Work out the finished part from the listing and answer in its coordinate system (mm). A direction names the side the tool comes from. Round coordinates to 2 decimals unless told otherwise and drop trailing zeros. Order: outer loops, then holes, each group sorted by start corner. A loop starts at its lowest first (then second) coordinate and runs counter-clockwise, first axis right, second up. Notation, with made-up numbers: (85.5, 23.5) -> (102.5, 23.5) arc R13 cw to (102.5, 43.5) -> close; hole circle Ø3 at (-38, 62.25). An arc over 180 degrees is marked (long way). Use a Markdown table: item, result. Add a question column.
Item 1: Find the intervals of material crossed by L1, parallel to Z at x = -2, y = 1.5; L2, parallel to X at y = -2.25, z = 21.5; L3, parallel to Y at x = -2, z = 27, in increasing order. Write a range as [from, to].
Item 2: A tool of negligible diameter and unlimited length cuts with its end or side. For faces 1 (the flat face through (-1.6, -1.4, 0)), 2 (the flat face through (-3.919, 0, 15)), 3 (the cylindrical face through (0.512, 0.583, 32.958)), from which of +Z, -Z, +X, -X, +Y, -Y can it reach the whole face along a straight path? Write none if from no direction.
Item 3: A cutting plane is placed at B-B, the plane y = -0.75. Determine the outline of the cut face in (x, z).
Item 4: A cutting plane is placed at C-C, the plane x = -1.5. Determine the outline of the cut face in (y, z), plus the area to 3 significant figures.
Item 5: A cutting plane is placed at D-D, the plane y = 2.25. Determine the outline of the cut face in (x, z), plus the area to 3 significant figures.
Item 6: A cutting plane is placed at A-A, the plane z = 3. Determine the outline of the cut face in (x, y).
from build123d import *

# Parameters (mm, degrees)
BOSS_EXTRUDE1_DEPTH = 30
SKETCH2_R           = 1.5
BOSS_EXTRUDE2_DEPTH = 6
SKETCH3_R           = 1.5
BOSS_EXTRUDE3_DEPTH = 6


with BuildPart() as part:
    # Sketch1 → Boss-Extrude1 (new body)
    with BuildSketch(Plane.XY):
        Polygon((-0.918598934, -3.331524887), (2.081401066, -1.599474079), (2.081401066, 1.864627536), (-0.918598934, 3.596678344), (-3.918598934, 1.864627536), (-3.918598934, -1.599474079), align=None)
    extrude(amount=BOSS_EXTRUDE1_DEPTH)

    # Sketch2 → Boss-Extrude2 (add)
    with BuildSketch(Plane.XY.offset(30)):
        with Locations((-0.918598934, 0.132576728)):
            Circle(SKETCH2_R)
    extrude(amount=BOSS_EXTRUDE2_DEPTH)

    # Sketch3 → Boss-Extrude3 (add)
    with BuildSketch(Plane(origin=(0, 0, 0), x_dir=(-1, 0, 0), z_dir=(0, 0, -1))):
        with Locations((0.918598934, 0.132576728)):
            Circle(SKETCH3_R)
    extrude(amount=BOSS_EXTRUDE3_DEPTH)


solid = part.part
Reported:
| question | item | result |
|---|---|---|
| 1 | L1 | [0, 30] |
| 1 | L2 | [-2.79, 0.95] |
| 1 | L3 | [-2.71, 2.97] |
| 2 | face 1 | -Z |
| 2 | face 2 | +Z, -Z, -X, +Y, -Y |
| 2 | face 3 | +Z |
| 3 | outline | (-3.92, 0) -> (-2.13, 0) -> (-2.13, -6) -> (0.29, -6) -> (0.29, 0) -> (2.08, 0) -> (2.08, 30) -> (0.29, 30) -> (0.29, 36) -> (-2.13, 36) -> (-2.13, 30) -> (-3.92, 30) -> close |
| 4 | outline | (-3, 0) -> (-1.25, 0) -> (-1.25, -6) -> (1.52, -6) -> (1.52, 0) -> (3.26, 0) -> (3.26, 30) -> (1.52, 30) -> (1.52, 36) -> (-1.25, 36) -> (-1.25, 30) -> (-3, 30) -> close |
| 4 | area | 221 mm² |
| 5 | outline | (-3.25, 0) -> (1.41, 0) -> (1.41, 30) -> (-3.25, 30) -> close |
| 5 | area | 140 mm² |
| 6 | outline | (-3.92, -1.6) -> (-0.92, -3.33) -> (2.08, -1.6) -> (2.08, 1.86) -> (-0.92, 3.6) -> (-3.92, 1.86) -> close |
